Build history of the part. All positions in model axes, mm. A direction names the side the tool comes from. Round coordinates to 2 decimals unless told otherwise and drop trailing zeros. Write each loop counter-clockwise with the first axis right and the second up, starting at its lowest first coordinate (ties: lowest second). Pieces come first, ordered by that corner, then holes. Notation, with made-up numbers: (85, 80.5) -> (108, 80.5) arc R25 cw to (108, 96.5) -> close; hole circle Ø5 at (-27, 20). An arc over 180 degrees is marked (long way). Return JSON: item names as keys, results as strings.
from build123d import *

# Parameters (mm, degrees)
BASE_FLANGE1_DEPTH            = 1.7366
EDGE_FLANGE1_START            = -115.730831119
EDGE_FLANGE1_DEPTH            = 204.671095583
EDGE_FLANGE1_2_DEPTH          = 0.8683
EDGE_FLANGE1_START_2          = 88.594139894
EDGE_FLANGE1_3_DEPTH          = 0.34612457
EDGE_FLANGE1_START_3          = -114.862531119
EDGE_FLANGE1_4_DEPTH          = 203.456671013
EDGE_FLANGE1_5_OUTLINE_W      = 29.4634
EDGE_FLANGE1_5_OUTLINE_H      = 1.7366
EDGE_FLANGE1_5_DEPTH          = 0.405860106
EDGE_FLANGE2_STRIP_W          = 8.4196
EDGE_FLANGE2_STRIP_H          = 1.7366
EDGE_FLANGE2_STRIP_CUT_DEPTH  = 203.662531119
EDGE_FLANGE2_RELIEF_W         = 9.2879
EDGE_FLANGE2_RELIEF_H         = 0.8683
EDGE_FLANGE2_RELIEF_CUT_DEPTH = 1.7366
EDGE_FLANGE2_DEPTH            = 203.662531119


# Read off the part's stored shape, not the designer's step: Edge-Flange1
# Sheet-metal steps are written as plain solids
with BuildPart() as part:
    # Sketch1 → Base-Flange1 (new body)
    with BuildSketch(Plane(origin=(0, 0, 0), x_dir=(0, 0, -1), z_dir=(1, 0, 0))):
        Polygon((2.253419205, 116.937468881), (-9.259888049, 92.904226435), (-12.275167803, 87.656070952), (-12.429418016, 87.67778326), (-15.116149142, 88.940264464), (-15.116149142, -117.062531119), (15.1, -117.062531119), (15.1, 116.937468881), align=None)
    extrude(amount=-BASE_FLANGE1_DEPTH)

    # Edge-Flange1 outline → Edge-Flange1 (cut)
    with BuildSketch(Plane(origin=(0, 0, 0), x_dir=(1, 0, 0), z_dir=(0, 1, 0)).offset(EDGE_FLANGE1_START)):
        with BuildLine():
            Line((0, -15.116149142), (0, -14.379549142))
            ThreePointArc((0, -14.379549142), (-0.02822066, -14.752100167), (-0.112238611, -15.116149142))
            Line((-0.112238611, -15.116149142), (0, -15.116149142))
        make_face()
    extrude(amount=EDGE_FLANGE1_DEPTH, mode=Mode.SUBTRACT)

    # Edge-Flange1 2 outline → Edge-Flange1 2 (cut)
    with BuildSketch(Plane(origin=(0, 0, 0), x_dir=(1, 0, 0), z_dir=(0, 1, 0)).offset(EDGE_FLANGE1_START)):
        with BuildLine():
            Line((0, -13.511249142), (-1.7366, -13.511249142))
            Line((-1.7366, -13.511249142), (-1.7366, -15.116149142))
            Line((-1.7366, -15.116149142), (-0.112238611, -15.116149142))
            ThreePointArc((-0.112238611, -15.116149142), (-0.02822066, -14.752100167), (0, -14.379549142))
            Line((0, -14.379549142), (0, -13.511249142))
        make_face()
    extrude(amount=EDGE_FLANGE1_2_DEPTH, mode=Mode.SUBTRACT)

    # Edge-Flange1 3 outline → Edge-Flange1 3 (cut)
    with BuildSketch(Plane(origin=(0, 0, 0), x_dir=(1, 0, 0), z_dir=(0, 1, 0)).offset(EDGE_FLANGE1_START_2)):
        with BuildLine():
            Line((0, -13.511249142), (-1.7366, -13.511249142))
            Line((-1.7366, -13.511249142), (-1.7366, -15.116149142))
            Line((-1.7366, -15.116149142), (-0.112238611, -15.116149142))
            ThreePointArc((-0.112238611, -15.116149142), (-0.02822066, -14.752100167), (0, -14.379549142))
            Line((0, -14.379549142), (0, -13.511249142))
        make_face()
    extrude(amount=EDGE_FLANGE1_3_DEPTH, mode=Mode.SUBTRACT)

    # Edge-Flange1 4 outline → Edge-Flange1 4 (add)
    with BuildSketch(Plane(origin=(0, 0, 0), x_dir=(1, 0, 0), z_dir=(0, 1, 0)).offset(EDGE_FLANGE1_START_3)):
        with BuildLine():
            Line((-1.7366, -15.116149142), (-1.7366, -14.379549142))
            ThreePointArc((-1.7366, -14.379549142), (-1.952345145, -14.900403997), (-2.4732, -15.116149142))
            Line((-2.4732, -15.116149142), (-31.9366, -15.116149142))
            Line((-31.9366, -15.116149142), (-31.9366, -16.852749142))
            Line((-31.9366, -16.852749142), (-2.4732, -16.852749142))
            ThreePointArc((-2.4732, -16.852749142), (-1.007771885, -16.371843969), (-0.112238611, -15.116149142))
            Line((-0.112238611, -15.116149142), (-1.7366, -15.116149142))
        make_face()
    extrude(amount=EDGE_FLANGE1_4_DEPTH)

    # Edge-Flange1 5 outline → Edge-Flange1 5 (add)
    with BuildSketch(Plane(origin=(0, 0, 0), x_dir=(1, 0, 0), z_dir=(0, 1, 0)).offset(EDGE_FLANGE1_START_2)):
        with Locations((-17.2049, -15.984449142)):
            Rectangle(EDGE_FLANGE1_5_OUTLINE_W, EDGE_FLANGE1_5_OUTLINE_H)
    extrude(amount=EDGE_FLANGE1_5_DEPTH)

    # Edge-Flange2 strip (across the edge) → Edge-Flange2 strip cut (cut)
    with BuildSketch(Plane(origin=(-31.9366, 89, 16.852749142), x_dir=(1, 0, 0), z_dir=(0, -1, 0))):
        with Locations((-3.4732, -0.8683)):
            Rectangle(EDGE_FLANGE2_STRIP_W, EDGE_FLANGE2_STRIP_H)
    extrude(amount=EDGE_FLANGE2_STRIP_CUT_DEPTH, mode=Mode.SUBTRACT)

    # Edge-Flange2 relief (on the sheet) → Edge-Flange2 relief cut (cut)
    with BuildSketch(Plane(origin=(-31.2, 89, 16.852749142), x_dir=(1, 0, 0), z_dir=(0, 0, 1))):
        with Locations((-3.77565, -204.096681119)):
            Rectangle(EDGE_FLANGE2_RELIEF_W, EDGE_FLANGE2_RELIEF_H)
    extrude(amount=-EDGE_FLANGE2_RELIEF_CUT_DEPTH, mode=Mode.SUBTRACT)

    # Edge-Flange2 section (across the edge) → Edge-Flange2 (add)
    with BuildSketch(Plane(origin=(-31.9366, 89, 16.852749142), x_dir=(1, 0, 0), z_dir=(0, -1, 0))):
        with BuildLine():
            Line((-1.7366, 0.7366), (-1.7366, 30.2))
            Line((-1.7366, 30.2), (0, 30.2))
            Line((0, 30.2), (0, 0.7366))
            ThreePointArc((0, 0.7366), (0.215745145, 0.215745145), (0.7366, 0))
            Line((0.7366, 0), (0.7366, -1.7366))
            ThreePointArc((0.7366, -1.7366), (-1.012216491, -1.012216491), (-1.7366, 0.7366))
        make_face()
    extrude(amount=EDGE_FLANGE2_DEPTH)


solid = part.part
Q1. Pin check, flat tips, straight feed: pin 1 Ø1 at (x, y) = (-1, -115.5) entering from +Z; pin 2 Ø2.5 at (x, z) = (-1, 16) entering from +Y; pin 3 Ø3.5 at (x, z) = (-9.5, 14.5) entering from -Y; pin 4 Ø12 at (x, z) = (-23.5, 24) entering from +Y. Stop position of each tip, or through.
Verdict:
{"pin 1": "stops at z = 15.12", "pin 2": "stops at y = 88.59", "pin 3": "stops at y = -114.86", "pin 4": "passes through"}
Q2. Saw through at A-A on y = -101. List the corners of the cut face in (x, z), then the cut area to 3 significant figures.
Verdict:
{"outline": "(-33.67, 17.59) arc R2.47 ccw to (-31.2, 15.12) -> (-2.47, 15.12) arc R0.74 cw to (-1.74, 14.38) -> (-1.74, -15.1) -> (0, -15.1) -> (0, 14.38) arc R2.47 ccw to (-2.47, 16.85) -> (-31.2, 16.85) arc R0.74 cw to (-31.94, 17.59) -> (-31.94, 47.05) -> (-33.67, 47.05) -> close", "area": "161 mm²"}
Q3. 3-axis set-ups, long thin cutter, end or side, ignore diameter. For faces 1 (the flat face through (-31.937, -11, 33)), 2 (the flat face through (-17, -14, 15.116)), 3 (the flat face through (-33, 89, 24)): which of +Z, -Z, +X, -X, +Y, -Y reach the whole face in a straight line?
Verdict:
{"face 1": "+Z, +X, +Y, -Y", "face 2": "-Z, -X, +Y, -Y", "face 3": "+Z, -Z, +X, -X, +Y"}
Q4. Wall check: L1, parallel to X at y = -69, z = 24.5; L2, parallel to Z at x = -10.5, y = 67.5; L3, parallel to X at y = 5.5, z = 3.5. Give the ranges that are in metal, low to high.
Verdict:
{"L1": "x = -33.67 to -31.94", "L2": "z = 15.12 to 16.85", "L3": "x = -1.74 to 0"}
Q5. Saw through at B-B on x = -26. List the corners of the cut face in (y, z).
Verdict:
{"outline": "(-114.86, 15.12) -> (89, 15.12) -> (89, 16.85) -> (-114.86, 16.85) -> close"}
Q6. Saw through at C-C on z = -8. List the corners of the cut face in (x, y), then the cut area to 3 significant figures.
Verdict:
{"outline": "(-1.74, -117.06) -> (0, -117.06) -> (0, 116.94) -> (-1.74, 116.94) -> close", "area": "406 mm²"}
